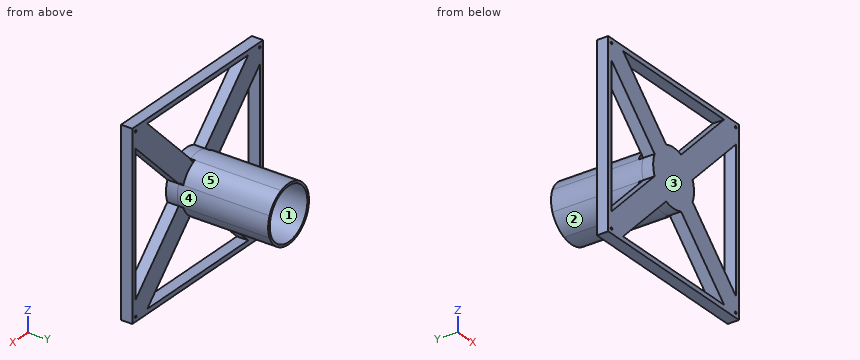
Autodesk Inventor part; units mm, degrees
ref_plane "YZ Plane" through (0, 0, 0) normal (1, 0, 0) x (0, 1, 0)
ref_plane "XZ Plane" through (0, 0, 0) normal (0, 1, 0) x (-1, 0, 0)
ref_plane "XY Plane" through (0, 0, 0) normal (0, 0, 1) x (1, 0, 0)
sketch "Sketch1" plane through (0, 0, 0) normal (0, 1, 0) x (-1, 0, 0)
  line L0 (-40, 40) -> (-40, -40)
  line L1 (-40, -40) -> (40, -40)
  line L2 (40, -40) -> (40, 40)
  line L3 (40, 40) -> (-40, 40)
  line L4 (18.0792, 11.0081) -> (40, 32.9289)
  line L5 (11.6365, -4.5654) -> (40, -32.9289)
  line L6 (32.9289, -40) -> (4.5654, -11.6365)
  line L7 (-4.5654, 11.6365) -> (-32.9289, 40)
  line L8 (-11.6365, 4.5654) -> (-40, 32.9289)
  line L9 (32.9289, 40) -> (4.5654, 11.6365)
  line L10 (-11.6365, -4.5654) -> (-40, -32.9289)
  line L11 (-3.5355, 3.5355) -> (0, 0) construction
  line L12 (18.0792, 11.0081) -> (11.6365, 4.5654)
  line L13 (-4.5654, -11.6365) -> (-32.9289, -40)
  line L14 (30.8898, 37.9609) -> (-30.8898, 37.9609)
  line L15 (38, 30.9289) -> (38, -30.9289)
  line L16 (30.8898, -37.9609) -> (-30.8898, -37.9609)
  line L17 (-38.0969, -31.0259) -> (-38.0969, 31.0259)
  circle A0 centre (0, 0) radius 12.5
  point P0 (0, 0)
  dimension "d8" = 25
  dimension "d0" = 80
  dimension "d1" = 80
  dimension "d3" = 10
  dimension "d4" = 10
  dimension "d5" = 10
  dimension "d6" = 10
  dimension "d7" = 2
  dimension "d9" = 7.0711
  dimension "d10" = 7.0711
  dimension "d11" = 7.0711
  dimension "d12" = 7.0711
  dimension "d13" = 7.0711
  dimension "d14" = 7.0711
  dimension "d15" = 7.0711
extrude "Extrusion1" add sketch "Sketch1" along normal blind 5 contours L3 L7 A0 L8 L0 | L8 L17 L10 L0 | L3 L9 L14 L7 | L10 A0 L13 L1 L0 | L3 L2 L4 L12 A0 L9 | A0 | L13 L16 L6 L1 | L2 L5 L15 L4 | L6 A0 L5 L2 L1
sketch "Sketch2" plane through (0, 5, 0) normal (0, 1, 0) x (1, 0, 0)
  line L0 (-11.6365, -4.5654) -> (-38, -30.9289)
  line L1 (-38, -30.9289) -> (-38, 30.9289)
  line L2 (-38, 30.9289) -> (-11.6365, 4.5654)
  arc A0 (-11.6365, 4.5654) -> (-11.6365, -4.5654) centre (0, 0) ccw
  line L3 (-4.5654, 11.6365) -> (-30.8898, 37.9609)
  line L4 (-30.8898, 37.9609) -> (30.8898, 37.9609)
  line L5 (30.8898, 37.9609) -> (4.5654, 11.6365)
  arc A1 (4.5654, 11.6365) -> (-4.5654, 11.6365) centre (0, 0) ccw
  line L6 (11.6365, 4.5654) -> (38.0969, 31.0259)
  line L7 (38.0969, 31.0259) -> (38.0969, -31.0259)
  line L8 (38.0969, -31.0259) -> (11.6365, -4.5654)
  arc A2 (11.6365, -4.5654) -> (11.6365, 4.5654) centre (0, 0) ccw
  arc A3 (-4.5654, -11.6365) -> (4.5654, -11.6365) centre (0, 0) ccw
  line L9 (4.5654, -11.6365) -> (30.8898, -37.9609)
  line L10 (30.8898, -37.9609) -> (-30.8898, -37.9609)
  line L11 (-30.8898, -37.9609) -> (-4.5654, -11.6365)
  line L12 (-40, 40) -> (-40, -40)
  line L13 (-40, -40) -> (40, -40)
  line L14 (40, -40) -> (40, 40)
  line L15 (40, 40) -> (-40, 40)
  circle A4 centre (0, 0) radius 12.5
  point P0 (0, 0)
extrude "Extrusion2" add sketch "Sketch2" along normal blind 40 contours A0 A4 A1 A2 A3
sketch "Sketch3" plane through (0, 45, 0) normal (0, 1, 0) x (1, 0, 0)
  circle A0 centre (0, 0) radius 11.5
  circle A1 centre (0, 0) radius 12.5
  dimension "d20" = 1
sketch "Sketch4" plane through (0, 5, 0) normal (0, 1, 0) x (1, 0, 0)
  line L0 (-40, 40) -> (-40, -40)
  line L1 (-40, -40) -> (40, -40)
  line L2 (40, -40) -> (40, 40)
  line L3 (40, 40) -> (-40, 40)
  arc A0 (-4.5654, 11.6365) -> (-11.6365, 4.5654) centre (0, 0) ccw
  line L4 (-4.5654, 11.6365) -> (-30.8898, 37.9609)
  line L5 (-30.8898, 37.9609) -> (30.8898, 37.9609)
  line L6 (30.8898, 37.9609) -> (4.5654, 11.6365)
  arc A1 (11.6365, 4.5654) -> (4.5654, 11.6365) centre (0, 0) ccw
  line L7 (11.6365, 4.5654) -> (38.0969, 31.0259)
  line L8 (38.0969, 31.0259) -> (38.0969, -31.0259)
  line L9 (38.0969, -31.0259) -> (11.6365, -4.5654)
  arc A2 (4.5654, -11.6365) -> (11.6365, -4.5654) centre (0, 0) ccw
  line L10 (4.5654, -11.6365) -> (30.8898, -37.9609)
  line L11 (30.8898, -37.9609) -> (-30.8898, -37.9609)
  line L12 (-30.8898, -37.9609) -> (-4.5654, -11.6365)
  arc A3 (-11.6365, -4.5654) -> (-4.5654, -11.6365) centre (0, 0) ccw
  line L13 (-11.6365, -4.5654) -> (-38, -30.9289)
  line L14 (-38, -30.9289) -> (-38, 30.9289)
  line L15 (-38, 30.9289) -> (-11.6365, 4.5654)
  line L16 (40, -40) -> (40, 40) construction
  line L17 (-40, 40) -> (40, -40) construction
  line L18 (40, -40) -> (-40, -40) construction
  line L19 (-40, -40) -> (40, 40) construction
  circle A4 centre (-38, 38) radius 1 construction
  circle A5 centre (-38, 38) radius 0.5
  line L20 (0, 42.5654) -> (0, -45.1181) construction
  line L21 (45.7517, 0) -> (-46.765, 0) construction
  circle A6 centre (38, 38) radius 0.5
  circle A7 centre (38, -38) radius 0.5
  circle A8 centre (-38, -38) radius 0.5
  point P0 (0, 0)
  dimension "d21" = 2
  dimension "d22" = 1
extrude "Extrusion3" cut sketch "Sketch4" against normal blind 40 contours A5 | A6 | A7 | A8
sketch "Sketch5" plane through (0, 0, 0) normal (1, 0, 0) x (0, 1, 0)
  line L0 (0, -12.5) -> (45, -12.5)
  line L1 (5, -37.9609) -> (5, -11.6365)
  line L2 (0, -37.9609) -> (0, -11.6365)
  line L3 (0, -11.6365) -> (5, -11.6365)
  line L4 (0, -31.0259) -> (5, -31.0259)
  line L5 (5, -4.5654) -> (5, -31.0259)
  line L6 (0, -4.5654) -> (5, -4.5654)
  line L7 (0, -4.5654) -> (0, -31.0259)
  line L8 (0, 31.0259) -> (5, 31.0259)
  line L9 (0, 31.0259) -> (0, 4.5654)
  line L10 (0, 4.5654) -> (5, 4.5654)
  line L11 (5, 31.0259) -> (5, 4.5654)
  line L12 (5, 11.6365) -> (5, 4.5654)
  line L13 (0, 12.5) -> (45, 12.5)
  line L14 (5, -31.0259) -> (5, 31.0259)
  line L15 (5, 40) -> (5, -40) construction
  line L16 (5, -12.5) -> (7, -12.5) construction
  line L17 (7, -12.5) -> (7, 12.5) construction
  line L18 (7, -10.5) -> (5, -10.5)
  line L19 (7, 10.5) -> (5, 10.5)
  line L20 (7, -10.5) -> (7, 10.5)
  line L21 (5, -10.5) -> (5, 10.5)
  line L22 (7, 0) -> (5, 0)
  line L23 (-9, 0) -> (54, 0)
  point P0 (0, 0)
  dimension "d25" = 2
  dimension "d26" = 2
  dimension "d27" = 2
revolve "Revolution1" cut sketch "Sketch5" angle 360 about axis through (0, -10, 0) along (0, 1, 0) contours L5 L14 L22 L20 L18
sketch "Sketch6" plane through (0, 5, 0) normal (0, 1, 0) x (1, 0, 0)
  circle A0 centre (0, 0) radius 12.5
  circle A1 centre (0, 0) radius 10.0217
  line L0 (11.6365, -4.5654) -> (0, 0)
  line L1 (0, 0) -> (4.6076, -11.6198)
  arc A2 (-4.5654, -11.6365) -> (4.5654, -11.6365) centre (0, 0) ccw
  line L2 (0, 0) -> (-4.5654, -11.6365)
  line L3 (-11.6365, -4.5654) -> (-38, -30.9289)
  line L4 (0, 0) -> (-11.6365, -4.5654)
  arc A3 (11.6365, -4.5654) -> (11.6365, 4.5654) centre (0, 0) ccw
  line L5 (0, 0) -> (11.6365, 4.5654)
  line L6 (11.6365, 4.5654) -> (0, 0)
  line L7 (0, 0) -> (4.5654, 11.6365)
  line L8 (0, 0) -> (-4.5654, 11.6365)
  line L9 (0, 0) -> (-11.6365, 4.5654)
extrude "Extrusion4" cut sketch "Sketch6" along normal blind 2 contours A0 L1 A1 L0 | A1 L1 L0 | L8 A1 L9 A0 | L9 A1 L8
sketch "Sketch7" plane through (0, 5, 0) normal (0, 1, 0) x (1, 0, 0)
  arc A0 (11.6365, -4.5654) -> (11.6365, 4.5654) centre (0, 0) ccw
  arc A1 (4.5654, -11.6365) -> (11.6365, -4.5654) centre (0, 0) ccw
  arc A2 (-11.6365, -4.5654) -> (-4.5654, -11.6365) centre (0, 0) ccw
  arc A3 (11.6365, 4.5654) -> (4.5654, 11.6365) centre (0, 0) ccw
  arc A4 (-4.5654, 11.6365) -> (-11.6365, 4.5654) centre (0, 0) ccw
  line L0 (11.6365, -4.5654) -> (8.3603, -3.28)
  line L1 (-8.3603, 3.28) -> (-11.6365, 4.5654)
  line L2 (4.5654, -11.6365) -> (3.28, -8.3603)
  line L3 (-3.28, 8.3603) -> (-4.5654, 11.6365)
  line L4 (-4.5654, -11.6365) -> (-3.28, -8.3603)
  line L5 (3.28, 8.3603) -> (4.5654, 11.6365)
  line L6 (-11.6365, -4.5654) -> (-8.3603, -3.28)
  line L7 (8.3603, 3.28) -> (11.6365, 4.5654)
  arc A5 (3.28, -8.3603) -> (8.3603, -3.28) centre (0, 0) ccw
  arc A6 (-8.3603, -3.28) -> (-3.28, -8.3603) centre (0, 0) ccw
  arc A7 (8.3603, 3.28) -> (3.28, 8.3603) centre (0, 0) ccw
  arc A8 (-3.28, 8.3603) -> (-8.3603, 3.28) centre (0, 0) ccw
  dimension "d31" = 8.9807
  dimension "d32" = 3.2761
  dimension "d33" = 3.2761
  dimension "d34" = 3.2761
extrude "Extrusion5" cut sketch "Sketch7" along normal blind 2
extrude "Extrusion6" cut sketch "Sketch3" against normal blind 40 contours A0
sketch "Sketch8" plane through (0, 45, 0) normal (0, 1, 0) x (1, 0, 0)
  point P0 (0, 0)
properties part number "Motor housing for Lifting Platform"
Here's how the part is built. I have some questions about the finished solid (model axes, mm). Face numbers are marked on the shaded views. A direction names the side the tool comes from. Round coordinates to 2 decimals unless told otherwise and drop trailing zeros. Order: outer loops, then holes, each group sorted by start corner. A loop starts at its lowest first (then second) coordinate and runs counter-clockwise, first axis right, second up. Notation, with made-up numbers: M 9.5,59 L 52.5,59 A24 cw 52.5,85 Z; hole C -38.75,-9 d5. An arc over 180 degrees is marked long. Use CSV: the item, a comma, the result in double quotes.
1) I want a section at D-D (x = -33). List the corners of the cut face in (y, z) for me.
Taken from the geometry:
outline,"M 0,-40 L 5,-40 L 5,-25.93 L 0,-25.93 Z; M 0,25.93 L 5,25.93 L 5,40 L 0,40 Z"
2) I'm going to push flat-ended pins straight in: P1, Ø1, axis at x = 10.5, y = 30, coming from the -Z side; P2, Ø18.5, axis at x = 0, z = 0, coming from the -Y side; P3, Ø3, axis at x = 14.5, z = -23, coming from the +Y side; P4, Ø6, axis at x = 10.5, y = 32, coming from the -Z side. Where does each tip first touch, or does it pass through?
Taken from the geometry:
P1,"z = -7.5"
P2,"y = 0"
P3,"y = 5"
P4,"z = -10"
3) If we mould it in two halves opening along X, with no side actions, what happens to the marked faces 1, 2 and 3? For each: pulls with the +X half, pulls with the -X half, needs draft (parallel to the pull), parting line crosses it, or undercut.
Taken from the geometry:
face 1,"undercut"
face 2,"pulls with the -X half"
face 3,"needs draft"
4) I want a section at C-C (x = -6.5). List the corners of the cut face in (y, z) for me.
Taken from the geometry:
outline,"M 0,-40 L 5,-40 L 5,-37.96 L 0,-37.96 Z; M 0,-13.57 L 5,-13.57 L 5,13.57 L 0,13.57 Z; M 0,37.96 L 5,37.96 L 5,40 L 0,40 Z; M 7,-10.68 L 45,-10.68 L 45,-9.49 L 7,-9.49 Z; M 7,9.49 L 45,9.49 L 45,10.68 L 7,10.68 Z"
5) I want a section at B-B (y = 40.5). List the corners of the cut face in (x, z) for me, then the cut area to 3 significant figures.
Taken from the geometry:
outline,"M -11.64,-4.57 A12.5 ccw -4.57,-11.64 A12.5 ccw 4.57,-11.64 A12.5 ccw 11.64,-4.57 A12.5 ccw 11.64,4.57 A12.5 ccw 4.57,11.64 A12.5 ccw -4.57,11.64 A12.5 ccw -11.64,4.57 A12.5 ccw Z; hole C 0,0 d23"
area,"75.4 mm^2"
6) I want a section at A-A (z = 0). List the corners of the cut face in (x, y) for me, then the cut area to 3 significant figures.
Taken from the geometry:
outline,"M -40,0 L -38,0 L -38,5 L -40,5 Z; M -12.5,0 L 12.5,0 L 12.5,45 L 11.5,45 L 11.5,5 L -11.5,5 L -11.5,45 L -12.5,45 Z; M 38.1,0 L 40,0 L 40,5 L 38.1,5 Z"
area,"225 mm^2"
7) I need wall thicknesses on line 1 along X through (y, z) = (1.65, 38); line 2 along Z through (x, y) = (38, 1.8); line 3 along X through (y, z) = (29.5, -0.5). Which ranges of each line are inside material? Lowest first, please. Write a range as [from, to].
Taken from the geometry:
line 1,"[-40, -38.5], [-37.5, 37.5], [38.5, 40]"
line 2,"[-40, -38.5], [-37.5, -30.93], [30.93, 37.5], [38.5, 40]"
line 3,"[-12.49, -11.49], [11.49, 12.49]"
8) On a 3-axis mill with a long thin cutter (end or side, diameter ignored), from which of +Z, -Z, +X, -X, +Y, -Y can I reach the whole of each face in a straight line? I mean the marked faces 4 and 5. Say none if no direction works.
Taken from the geometry:
face 4,"+X, +Y, -Y"
face 5,"+Z, +X, +Y"
